CAD build for the part. Positions are in the model's coordinates, mm. Face numbers are marked on the shaded views. Round coordinates to 2 decimals unless told otherwise and drop trailing zeros. Write each loop counter-clockwise with the first axis right and the second up, starting at its lowest first coordinate (ties: lowest second). Pieces come first, ordered by that corner, then holes. Notation, with made-up numbers: (61, -25) -> (81, -25) arc R24 ccw to (81, -11) -> close; hole circle Ø8 at (4, 68.25). An arc over 180 degrees is marked (long way). Put each result on its own line as item: value. Start each with the question number.
1. Drill centre lines: line 1 (Y direction, x = -38, z = 32); line 2 (Y direction, x = 10, z = -40); line 3 (X direction, y = -86, z = 31). Where is each one in solid material? Low to high. Write a range as from..to.
2. Saw through at A-A on x = 38. List the corners of the cut face in (y, z), and give its area (3 significant figures).
3. Saw through at B-B on y = -13. List the corners of the cut face in (x, z).
4. Pull direction Z, two halves, no side cores. Call the marked faces 1, 2, 3 and 4: pulls with the +Z half, pulls with the -Z half, needs draft (parallel to the pull), parting line crosses it, or undercut.
5. Flat gauge pins, fed straight in: P1, Ø3, axis at x = -22, z = 4.5, coming from the -Y side; P2, Ø6, axis at y = -48, z = -14, coming from the -X side; P3, Ø1.5, axis at x = 5.5, y = -58, coming from the -Z side. Where does each tip first touch, or does it go through?
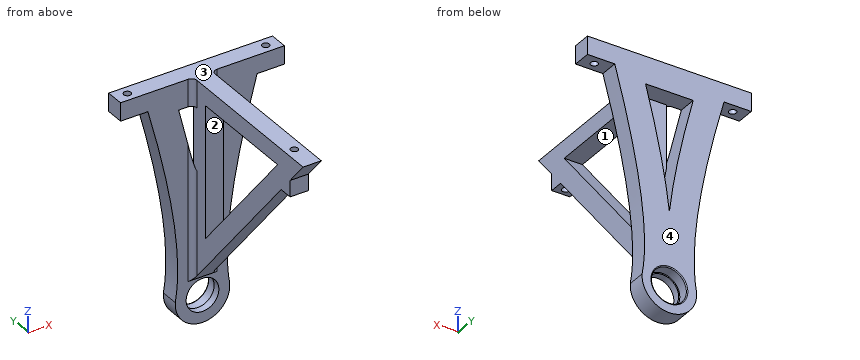
from build123d import *

# Parameters (mm, degrees)
EXTRUDE_1_DEPTH      = 10
SKETCH_2_R           = 9.65
CUT_EXTRUDE_1_DEPTH  = 6
SKETCH_3_R           = 9
CUT_EXTRUDE_2_DEPTH  = 108.971611223
SKETCH_4_R           = 2
CUT_EXTRUDE_3_DEPTH  = 134.22912608
FILLET_2_R           = 0.5
EXTRUDE_3_DEPTH      = 5
EXTRUDE_3_DEPTH_BACK = 5
FILLET_3_R           = 3
FILLET_4_R           = 3
FILLET_5_R           = 3
FILLET_6_R           = 3
SKETCH_8_W           = 10
SKETCH_8_H           = 8.119253015
EXTRUDE_5_DEPTH      = 22
SKETCH_7_R           = 2
CUT_EXTRUDE_4_DEPTH  = 170.615645405


with BuildPart() as part:
    # Эскиз1 → Бобышка-Вытянуть1 (new body)
    with BuildSketch(Plane(origin=(0, 0, 0), x_dir=(1, 0, 0), z_dir=(0, 1, 0))):
        with BuildLine():
            Line((-45, -37.036390428), (45, -37.036390428))
            Line((45, -37.036390428), (45, -27.036390428))
            Line((45, -27.036390428), (30, -27.036390428))
            add(Edge.make_bspline(
                [(30, -27.036390428), (8.982189831, 48.482679734), (14.96841635, 81.990721102)],
                knots=[0, 0, 0, 0.673052388, 0.673052388, 0.673052388], degree=2))
            ThreePointArc((14.96841635, 81.990721102), (0, 97.963609572), (-14.96841635, 81.990721102))
            add(Edge.make_bspline(
                [(-30, -27.036390428), (-8.982189831, 48.482679734), (-14.96841635, 81.990721102)],
                knots=[0, 0, 0, 0.673052388, 0.673052388, 0.673052388], degree=2))
            Line((-30, -27.036390428), (-45, -27.036390428))
            Line((-45, -27.036390428), (-45, -37.036390428))
        make_face()
        with BuildLine():
            Line((-13.093802095, -22.036390428), (13.093802095, -22.036390428))
            add(Edge.make_bspline(
                [(0, 42.892969081), (0.131197091, 41.727442037), (0.406798356, 39.416984329), (1.035729687, 34.652549779), (1.955297059, 28.529668977), (3.27425138, 20.876880517), (4.806507266, 12.923420182), (6.551708297, 4.662649881), (8.508532438, -3.905250597), (10.317434597, -11.311565536), (11.866516335, -17.379327452), (12.683259953, -20.491905055), (13.093802095, -22.036390428)],
                knots=[0.040117253, 0.040117253, 0.040117253, 0.040117253, 0.061247944, 0.082378635, 0.124640016, 0.166901397, 0.209162778, 0.251424159, 0.29368554, 0.335946921, 0.357077612, 0.378208302, 0.378208302, 0.378208302, 0.378208302], degree=3))
            add(Edge.make_bspline(
                [(-13.093802095, -22.036390428), (-12.683259953, -20.491905055), (-11.866516335, -17.379327452), (-10.317434597, -11.311565536), (-8.508532438, -3.905250597), (-6.551708297, 4.662649881), (-4.806507266, 12.923420182), (-3.27425138, 20.876880517), (-1.955297059, 28.529668977), (-1.035729687, 34.652549779), (-0.406798356, 39.416984329), (-0.131197091, 41.727442037), (0, 42.892969081)],
                knots=[0.040117253, 0.040117253, 0.040117253, 0.040117253, 0.061247944, 0.082378635, 0.124640016, 0.166901397, 0.209162778, 0.251424159, 0.29368554, 0.335946921, 0.357077612, 0.378208302, 0.378208302, 0.378208302, 0.378208302], degree=3))
        make_face(mode=Mode.SUBTRACT)
    extrude(amount=EXTRUDE_1_DEPTH)

    # Эскиз2 → Вырез-Вытянуть1 (cut)
    with BuildSketch(Plane(origin=(0, 10, 0), x_dir=(1, 0, 0), z_dir=(0, 1, 0))):
        with Locations(Location((0, 82.963609572, 0), (0, 0, 270))):
            Circle(SKETCH_2_R)
    extrude(amount=-CUT_EXTRUDE_1_DEPTH, mode=Mode.SUBTRACT)

    # Эскиз3 → Вырез-Вытянуть2 (cut, through all)
    with BuildSketch(Plane(origin=(0, 4, 0), x_dir=(1, 0, 0), z_dir=(0, 1, 0))):
        with Locations(Location((0, 82.963609572, 0), (0, 0, 270))):
            Circle(SKETCH_3_R)
    extrude(amount=-CUT_EXTRUDE_2_DEPTH, mode=Mode.SUBTRACT)

    # Эскиз4 → Вырез-Вытянуть3 (cut, through all)
    with BuildSketch(Plane(origin=(0, 0, 27.036390428), x_dir=(-1, 0, 0), z_dir=(0, 0, -1))):
        with Locations((38, 5)):
            Circle(SKETCH_4_R)
        with Locations((-38, 5)):
            Circle(SKETCH_4_R)
    extrude(amount=-CUT_EXTRUDE_3_DEPTH, mode=Mode.SUBTRACT)

    # Скругление2
    fillet_2_edges = [part.edges().sort_by_distance(p)[0] for p in [
        (0, 10, -92.613609572),
    ]]
    fillet(fillet_2_edges, radius=FILLET_2_R)

    # Эскиз6 → Бобышка-Вытянуть3 (add, two sides)
    with BuildSketch(Plane(origin=(0, 0, 0), x_dir=(0, 0, -1), z_dir=(1, 0, 0))) as extrude_3_sk:
        Polygon((72.963609572, 0), (-37.036390428, 0), (-37.036390428, -92.300959429), align=None)
        Polygon((45.488835377, -10), (-27.036390428, -10), (-27.036390428, -70.855890224), align=None, mode=Mode.SUBTRACT)
    extrude(amount=EXTRUDE_3_DEPTH)
    extrude(extrude_3_sk.sketch, amount=-EXTRUDE_3_DEPTH_BACK)

    # Скругление3
    fillet_3_edges = [part.edges().sort_by_distance(p)[0] for p in [
        (5, 0, 29.536390428),
    ]]
    fillet(fillet_3_edges, radius=FILLET_3_R)

    # Скругление4
    fillet_4_edges = [part.edges().sort_by_distance(p)[0] for p in [
        (5, 0, -42.52878468),
    ]]
    fillet(fillet_4_edges, radius=FILLET_4_R)

    # Скругление5
    fillet_5_edges = [part.edges().sort_by_distance(p)[0] for p in [
        (-5, 0, -42.52878468),
    ]]
    fillet(fillet_5_edges, radius=FILLET_5_R)

    # Скругление6
    fillet_6_edges = [part.edges().sort_by_distance(p)[0] for p in [
        (-5, 0, 29.536390428),
    ]]
    fillet(fillet_6_edges, radius=FILLET_6_R)

    # Эскиз8 → Бобышка-Вытянуть5 (add)
    with BuildSketch(Plane.XY.offset(37.036390428)):
        with Locations((0, -77.30095943)):
            Rectangle(SKETCH_8_W, SKETCH_8_H)
    extrude(amount=-EXTRUDE_5_DEPTH)

    # Эскиз7 → Вырез-Вытянуть4 (cut, through all)
    with BuildSketch(Plane.XY.offset(37.036390428)):
        with Locations((0, -77.300959429)):
            Circle(SKETCH_7_R)
    extrude(amount=-CUT_EXTRUDE_4_DEPTH, mode=Mode.SUBTRACT)


solid = part.part
Return value:
1. line 1: y = 0..3, 7..10
1. line 2: y = 0..10
1. line 3: x = -5..5
2. outline: (0, 27.04) -> (3, 27.04) -> (3, 37.04) -> (0, 37.04) -> close; (7, 27.04) -> (10, 27.04) -> (10, 37.04) -> (7, 37.04) -> close
2. area: 60.0 mm^2
3. outline: (-5, -57.47) -> (5, -57.47) -> (5, -41.91) -> (-5, -41.91) -> close; (-5, 27.04) -> (5, 27.04) -> (5, 37.04) -> (-5, 37.04) -> close
4. face 1: undercut
4. face 2: undercut
4. face 3: pulls with the +Z half
4. face 4: needs draft
5. P1: stops at y = 0
5. P2: stops at x = -5
5. P3: stops at z = -4.51
